Model file for the job. Use its own axes, mm. A direction names the side the tool comes from. Coordinates: 2 decimals unless noted, no trailing zeros. Order: outer loops, then holes, each group sorted by start corner. A loop starts at its lowest first (then second) coordinate and runs counter-clockwise, first axis right, second up. Notation, with made-up numbers: (16, 61.5) -> (52, 61.5) arc R31 ccw to (52, 87.5) -> close; hole circle Ø9 at (58.25, 21). An arc over 180 degrees is marked (long way). Write item = value, one per line. Start each with the question number.
Q1. 3-axis set-ups, long thin cutter, end or side, ignore diameter. For faces 1 (the face through (-51, 84, 0)), 2 (the face through (35.3, 4.9, 15.5)), 3 (the face through (-2, 10, 12)): which of +Z, -Z, +X, -X, +Y, -Y reach the whole face in a straight line?
Q2. Wall check: line 1 (X direction, y = 5, z = 15); line 2 (X direction, y = 27.5, z = 12.5); line 3 (X direction, y = 142, z = 20). Give the ranges that are in metal, low to high. Write a range as from..to.
Q3. Flat gauge pins, fed straight in: pin 1 (12 mm diameter, centred on x = 39.5, z = 9.5, fed in from +Y); pin 2 (8 mm diameter, centred on x = 0.5, z = 9, fed in from +Y). Where does each tip first touch, or does it go through?
Q4. Cut at A-A, the plane z = 15. List the corners of the cut face in (x, y).
Q5. Cut at B-B, the plane z = 7. List the corners of the cut face in (x, y), plus the area to 3 significant figures.
Q6. Cut at D-D, the plane x = 23.5. List the corners of the cut face in (y, z).
Q7. Cut at C-C, the plane y = 166. List the corners of the cut face in (x, z), plus the area to 3 significant figures.
Q8. Mould opens along Y. For faces 4 (the face through (52.749, 70, 15)), 5 (the face through (-3, 0, 15)), 6 (the face through (47.42, 144.48, 15.21)), 7 (the face through (-2, 100, 25)) say: +Y half, -Y half, draft (parallel to the pull), parting line (faces both ways), or undercut.
from build123d import *

# Parameters (mm, degrees)
BOSS_EXTRUDE1_DEPTH        = 30
CUT_EXTRUDE1_DEPTH         = 25
F_5_0MM_DOWEL_HOLE2_REACH  = 221.224
F_5_0MM_DOWEL_HOLE2_BORE_R = 2.5
F_5_0MM_DOWEL_HOLE4_D      = 5


with BuildPart() as part:
    # Sketch1 → Boss-Extrude1 (new body)
    with BuildSketch(Plane.XY):
        with BuildLine():
            Line((-57.251461988, 0), (52.748538012, 0))
            Line((52.748538012, 0), (52.748538012, 142))
            ThreePointArc((52.748538012, 142), (-2.251461988, 197), (-57.251461988, 142))
            Line((-57.251461988, 142), (-57.251461988, 0))
        make_face()
    extrude(amount=BOSS_EXTRUDE1_DEPTH)

    # Sketch8 → Cut-Extrude1 (cut)
    with BuildSketch(Plane(origin=(0, 0, 0), x_dir=(-1, 0, 0), z_dir=(0, 0, -1))):
        with BuildLine():
            Line((-42.748538012, 10), (47.251461988, 10))
            Line((47.251461988, 10), (47.251461988, 142))
            ThreePointArc((47.251461988, 142), (2.251461988, 187), (-42.748538012, 142))
            Line((-42.748538012, 142), (-42.748538012, 10))
        make_face()
    extrude(amount=-CUT_EXTRUDE1_DEPTH, mode=Mode.SUBTRACT)

    # Ø5.0mm Dowel Hole2 bore (on position points) → Ø5.0mm Dowel Hole2 (cut, up to next)
    with BuildSketch(Plane(origin=(-42.251461988, 0, 15), x_dir=(0, 0, -1), z_dir=(0, -1, 0)), mode=Mode.PRIVATE) as f_5_0mm_dowel_hole2_sk1:
        Circle(F_5_0MM_DOWEL_HOLE2_BORE_R)
    f_5_0mm_dowel_hole2_tool1 = extrude(f_5_0mm_dowel_hole2_sk1.sketch, amount=-F_5_0MM_DOWEL_HOLE2_REACH, mode=Mode.PRIVATE) & part.part
    # Ø5.0mm Dowel Hole2 bore (on position points) → Ø5.0mm Dowel Hole2 (cut, up to next)
    with BuildSketch(Plane(origin=(-42.251461988, 0, 15), x_dir=(0, 0, -1), z_dir=(0, -1, 0)), mode=Mode.PRIVATE) as f_5_0mm_dowel_hole2_sk2:
        with Locations((0, 80)):
            Circle(F_5_0MM_DOWEL_HOLE2_BORE_R)
    f_5_0mm_dowel_hole2_tool2 = extrude(f_5_0mm_dowel_hole2_sk2.sketch, amount=-F_5_0MM_DOWEL_HOLE2_REACH, mode=Mode.PRIVATE) & part.part
    add(f_5_0mm_dowel_hole2_tool1.solids().sort_by_distance((-42.251462, 0, 15))[0], mode=Mode.SUBTRACT)
    add(f_5_0mm_dowel_hole2_tool2.solids().sort_by_distance((37.748538, 0, 15))[0], mode=Mode.SUBTRACT)

    # Ø5.0mm Dowel Hole4 (through all)
    with Locations(Plane(origin=(47.748538012, 142, 0), x_dir=(-1, 0, 0), z_dir=(0, 0, -1))):
        with Locations((0, 0), (100, 0)):
            Hole(F_5_0MM_DOWEL_HOLE4_D / 2)


solid = part.part
Here are the results:
q1.face_1 = -Z, +X, -X, +Y, -Y
q1.face_2 = -Y
q1.face_3 = -Z
q2.line_1 = -57.25..-44.75, -39.75..35.25, 40.25..52.75
q2.line_2 = -57.25..-47.25, 42.75..52.75
q2.line_3 = -57.25..-54.75, -49.75..-47.25, 42.75..45.25, 50.25..52.75
q3.pin_1 = 183.8
q3.pin_2 = 197
q4.outline = (-57.25, 0) -> (-44.75, 0) -> (-44.75, 10) -> (-47.25, 10) -> (-47.25, 142) arc R45 cw to (42.75, 142) -> (42.75, 10) -> (40.25, 10) -> (40.25, 0) -> (52.75, 0) -> (52.75, 142) arc R55 ccw to (-57.25, 142) -> close; (-39.75, 0) -> (35.25, 0) -> (35.25, 10) -> (-39.75, 10) -> close; hole circle Ø5 at (-52.25, 142); hole circle Ø5 at (47.75, 142)
q5.outline = (-57.25, 0) -> (52.75, 0) -> (52.75, 142) arc R55 ccw to (-57.25, 142) -> close; hole circle Ø5 at (-52.25, 142); hole (-47.25, 10) -> (42.75, 10) -> (42.75, 142) arc R45 ccw to (-47.25, 142) -> close; hole circle Ø5 at (47.75, 142)
q5.area = 5,270 mm²
q6.outline = (0, 0) -> (10, 0) -> (10, 25) -> (178.9, 25) -> (178.9, 0) -> (190.6, 0) -> (190.6, 30) -> (0, 30) -> close
q7.outline = (-51.74, 0) -> (-40.32, 0) -> (-40.32, 25) -> (35.81, 25) -> (35.81, 0) -> (47.24, 0) -> (47.24, 30) -> (-51.74, 30) -> close
q7.area = 1,070 mm²
q8.face_4 = draft
q8.face_5 = -Y half
q8.face_6 = undercut
q8.face_7 = undercut
